```python
from build123d import *

# Parameters (mm, degrees)
BOSS_EXTRUDE1_DEPTH            = 6
BOSS_EXTRUDE2_DEPTH            = 5
BOSS_EXTRUDE2_DEPTH_BACK       = 6
SKETCH2_R                      = 7.5
SKETCH3_R                      = 6
BOSS_EXTRUDE3_DEPTH            = 6
SKETCH4_R                      = 4.1
CUT_EXTRUDE1_DEPTH             = 14
M4_CLEARANCE_HOLE1_D           = 4.5
M4_CLEARANCE_HOLE1_CSINK_D     = 4.55
M4_CLEARANCE_HOLE1_CSINK_ANGLE = 90
FILLET4_R                      = 0.5


with BuildPart() as part:
    # Sketch1 → Boss-Extrude1 (new body)
    with BuildSketch(Plane.XY):
        with BuildLine():
            Line((17, 4), (0.996565203, 7.5))
            Line((0.996565203, 7.5), (-0.996565203, 7.5))
            Line((-0.996565203, 7.5), (-17, 4))
            ThreePointArc((-17, 4), (-21, 0), (-17, -4))
            Line((-17, -4), (-0.996565203, -7.5))
            Line((-0.996565203, -7.5), (0.996565203, -7.5))
            Line((0.996565203, -7.5), (17, -4))
            ThreePointArc((17, -4), (21, 0), (17, 4))
        make_face()
    extrude(amount=BOSS_EXTRUDE1_DEPTH)

    # Sketch2 → Boss-Extrude2 (add, two sides: drawn at the far end of the back side and taken through both)
    with BuildSketch(Plane.XY.offset(6).offset(-BOSS_EXTRUDE2_DEPTH_BACK)):
        Circle(SKETCH2_R)
    extrude(amount=BOSS_EXTRUDE2_DEPTH + BOSS_EXTRUDE2_DEPTH_BACK)

    # Sketch3 → Boss-Extrude3 (add)
    with BuildSketch(Plane.XY.offset(11)):
        Circle(SKETCH3_R)
    extrude(amount=BOSS_EXTRUDE3_DEPTH)

    # Sketch4 → Cut-Extrude1 (cut)
    with BuildSketch(Plane.XY.offset(17)):
        Circle(SKETCH4_R)
    extrude(amount=-CUT_EXTRUDE1_DEPTH, mode=Mode.SUBTRACT)

    # M4 Clearance Hole1 (through all)
    with Locations(Plane(origin=(17, 0, 6), x_dir=(1, 0, 0), z_dir=(0, 0, 1))):
        with Locations((0, 0), (-34, 0)):
            CounterSinkHole(M4_CLEARANCE_HOLE1_D / 2, M4_CLEARANCE_HOLE1_CSINK_D / 2, counter_sink_angle=M4_CLEARANCE_HOLE1_CSINK_ANGLE)

    # Fillet4
    # the kernel refuses this fillet: 0.5 mm, written as the material it takes off along each edge
    with BuildSketch(Plane(origin=(17, 0, 5.975), x_dir=(-1, 0, 0), z_dir=(0, -1, 0))) as fillet4_piece_1:
        with BuildLine():
            CenterArc((2.75, 0.13112495), FILLET4_R, 180, 18.194872339)
            Line((2.25, 0.13112495), (2.24, 0.13112495))
            Line((2.24, 0.13112495), (2.24, 0))
            Line((2.24, 0), (2.242928932, -0.007071068))
            ThreePointArc((2.242928932, -0.007071068), (2.255428932, -0.019571068), (2.2655, -0.028122499))
            Line((2.2655, -0.028122499), (2.275, -0.025))
        make_face()
    revolve(axis=Axis((17, 0, 5.975), (0, 0, -1)), mode=Mode.SUBTRACT)


solid = part.part
```
Can you work these out from the model? Positions are in its coordinate system, mm. A direction names the side the tool comes from. Round coordinates to 2 decimals unless told otherwise and drop trailing zeros. Loops run counter-clockwise (first coordinate to the right, second up) from the corner with the lowest first, then second, coordinate; pieces in that order, holes last.
Item 1: Suppose I cut it at D-D, the plane x = 2. Write out the boundary of the cut face in (y, z), then the cut area to 3 significant figures.
Item 2: Suppose I cut it at B-B, the plane y = 0. Write out the boundary of the cut face in (x, z) (3 decimals).
Item 3: Please list where these lines run through material, in increasing order: L1, parallel to Y at x = -17, z = 4.4; L2, parallel to Z at x = 9, y = 3; L3, parallel to Y at x = -0.5, z = 10.
Item 4: Suppose I cut it at C-C, the plane z = 1.5. Write out the boundary of the cut face in (x, y), then the cut area to 3 significant figures.
Item 5: If we mould it in two halves opening along X, with no side actions, what happens to faces 3 (the cylindrical face through (-0.534, 4.065, 10.098)), 4 (the flat face through (-9.11, -5.726, 2.958)), 5 (the cylindrical face through (-7.493, 0.33, 8.465)), 6 (the cylindrical face through (-19.146, 0.676, 2.946))? For each: +X half, -X half, draft (parallel to the pull), parting line (faces both ways), or undercut.
Item 6: Will these pins go through, and if not, where does the flat tip stop? pin 1 Ø8 at (y, z) = (3, 13) entering from +X; pin 2 Ø2 at (x, y) = (16.5, -5.5) entering from +Z; pin 3 Ø2 at (x, z) = (-4, 2) entering from +Y; pin 4 Ø4.5 at (x, y) = (8.5, -1) entering from +Z.
Item 7: Which directions (+Z, -Z, +X, -X, +Y, -Y) give clear straight access to the entire face, cutting with the end or side of a thin tool? Please do faces 1 (the flat face through (2, 6, 11)), 2 (the cylindrical face through (21, 0, 3)).
Item 8: Suppose I cut it at A-A, the plane z = 4.5. Write out the boundary of the cut face in (x, y).
Reported:
1. outline: (-7.28, 0) - (7.28, 0) - (7.28, 6) - (7.23, 6) - (7.23, 11) - (5.66, 11) - (5.66, 17) - (3.58, 17) - (3.58, 3) - (-3.58, 3) - (-3.58, 17) - (-5.66, 17) - (-5.66, 11) - (-7.23, 11) - (-7.23, 6) - (-7.28, 6) - close
1. area: 127 mm2
2. outline: (-21, 0) - (-19.25, 0) - (-19.25, 5.975) - (-19.275, 6) - (-21, 6) - close; (-14.75, 0) - (14.75, 0) - (14.75, 5.844) arc R0.5 ccw to (14.725, 6) - (7.5, 6) - (7.5, 11) - (6, 11) - (6, 17) - (4.1, 17) - (4.1, 3) - (-4.1, 3) - (-4.1, 17) - (-6, 17) - (-6, 11) - (-7.5, 11) - (-7.5, 6) - (-14.725, 6) - (-14.75, 5.975) - close; (19.25, 0) - (21, 0) - (21, 6) - (19.275, 6) arc R0.5 ccw to (19.25, 5.844) - close
3. L1: y = -4 to -2.25, 2.25 to 4
3. L2: z = 0 to 6
3. L3: y = -7.48 to -4.07, 4.07 to 7.48
4. outline: (-17, -4) - (-1, -7.5) - (1, -7.5) - (17, -4) arc R4 ccw to (17, 4) - (1, 7.5) - (-1, 7.5) - (-17, 4) arc R4 ccw to start; hole circle Ø4.5 at (-17, 0); hole circle Ø4.5 at (17, 0)
4. area: 416 mm2
5. face 3: undercut
5. face 4: -X half
5. face 5: parting line
5. face 6: undercut
6. pin 1: stops at x = 7.5
6. pin 2: passes through
6. pin 3: stops at y = 7.06
6. pin 4: stops at z = 11
7. face 1: +Z
7. face 2: +Z, -Z, +X
8. outline: (-17, -4) - (-1, -7.5) - (1, -7.5) - (17, -4) arc R4 ccw to (17, 4) - (1, 7.5) - (-1, 7.5) - (-17, 4) arc R4 ccw to start; hole circle Ø4.5 at (-17, 0); hole circle Ø8.2 at (0, 0); hole circle Ø4.5 at (17, 0)
